Could you check a few things on this drawing? It's one solid part, dimensions in mm from its lowest x, y, z. Coordinates: 2 decimals unless noted, no trailing zeros. Order: outer loops, then holes, each group sorted by start corner. A loop starts at its lowest first (then second) coordinate and runs counter-clockwise, first axis right, second up.
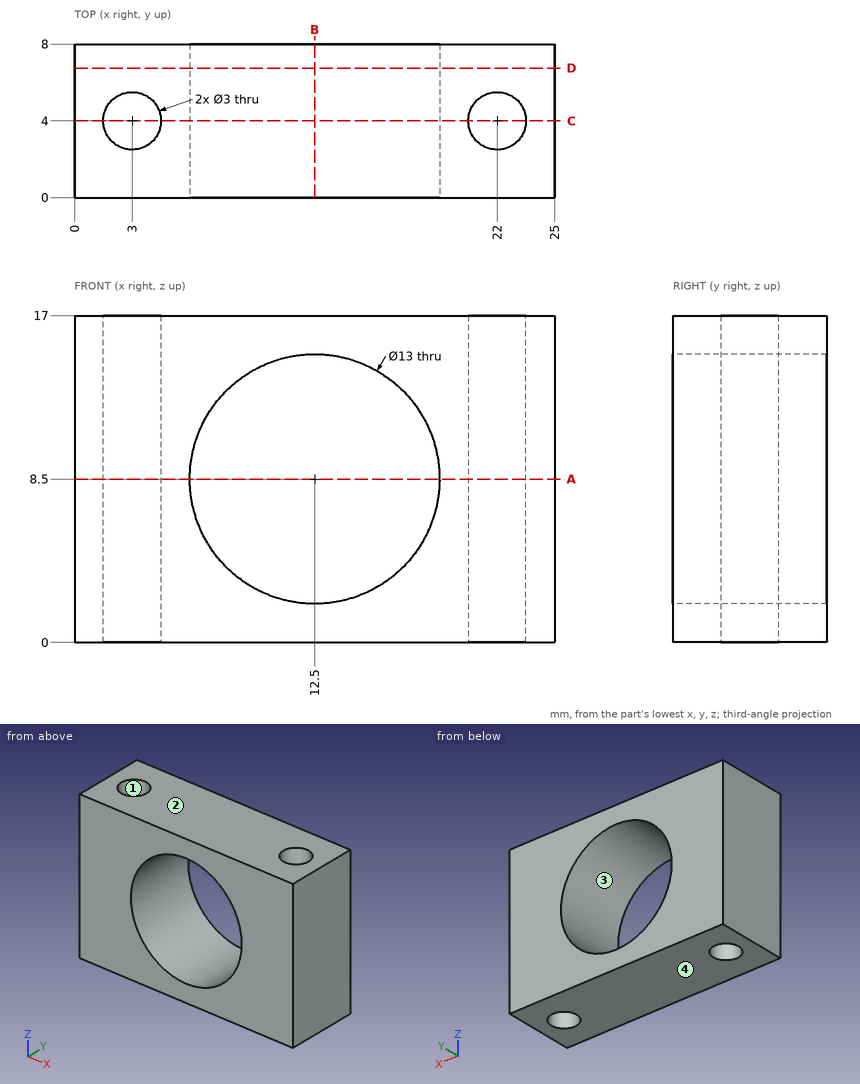
Q1. If we section it at B-B on x = 12.5: Write out the boundary of the cut face in (y, z), then the cut area to 3 significant figures.
Q2. Will this pin go through, and if not, where does the flat tip stop? pin 1 (4 mm diameter, centred on x = 22, y = 4, fed in from -Z).
Q3. If we section it at D-D on y = 6.75: Write out the boundary of the cut face in (x, z).
Q4. I need wall thicknesses on L1, parallel to X at y = 6, z = 8.5; L2, parallel to Y at x = 3, z = 5; L3, parallel to X at y = 3.5, z = 5. Which ranges of each line are inside material? Lowest first, please.
Q5. If we section it at C-C on y = 4: Write out the boundary of the cut face in (x, z), then the cut area to 3 significant figures.
Q6. If we section it at A-A on z = 8.5: Write out the boundary of the cut face in (x, y).
Q7. We'd pull the mould along Z, two halves only. Please class the marked faces 1, 2, 3 and 4: pulls with the +Z half, pulls with the -Z half, needs draft (parallel to the pull), parting line crosses it, or undercut.
Reply:
1. outline: (0, 0) - (8, 0) - (8, 2) - (0, 2) - close; (0, 15) - (8, 15) - (8, 17) - (0, 17) - close
1. area: 32.0 mm2
2. pin 1: stops at z = 0
3. outline: (0, 0) - (25, 0) - (25, 17) - (0, 17) - close; hole circle Ø13 at (12.5, 8.5)
4. L1: x = 0 to 6, 19 to 25
4. L2: y = 0 to 2.5, 5.5 to 8
4. L3: x = 0 to 1.59, 4.41 to 7.02, 17.98 to 20.59, 23.41 to 25
5. outline: (0, 0) - (1.5, 0) - (1.5, 17) - (0, 17) - close; (4.5, 0) - (20.5, 0) - (20.5, 17) - (4.5, 17) - close; (23.5, 0) - (25, 0) - (25, 17) - (23.5, 17) - close; hole circle Ø13 at (12.5, 8.5)
5. area: 190 mm2
6. outline: (0, 0) - (6, 0) - (6, 8) - (0, 8) - close; (19, 0) - (25, 0) - (25, 8) - (19, 8) - close; hole circle Ø3 at (3, 4); hole circle Ø3 at (22, 4)
7. face 1: needs draft
7. face 2: pulls with the +Z half
7. face 3: undercut
7. face 4: pulls with the -Z half
